from build123d import *

# Parameters (mm, degrees)
F0_R     = 2.794
F1_DEPTH = 2.38125


with BuildPart() as f1:
    # F0 (on Front) → F1 (new body, symmetric)
    with BuildSketch(Plane.XZ):
        with BuildLine():
            ThreePointArc((13.787585, 45.968807), (0, 53.975), (-13.787585, 45.968807))
            Line((-13.787585, 45.968807), (-36.430068, 6.295045))
            ThreePointArc((-36.430068, 6.295045), (-38.1, 0), (-36.430068, -6.295045))
            Line((-36.430068, -6.295045), (-13.787585, -45.968807))
            ThreePointArc((-13.787585, -45.968807), (0, -53.975), (13.787585, -45.968807))
            Line((13.787585, -45.968807), (36.430068, -6.295045))
            ThreePointArc((36.430068, -6.295045), (38.1, 0), (36.430068, 6.295045))
            Line((36.430068, 6.295045), (13.787585, 45.968807))
        make_face()
        with Locations((0, -44.45)):
            Circle(F0_R, mode=Mode.SUBTRACT)
        with Locations((0, 44.45)):
            Circle(F0_R, mode=Mode.SUBTRACT)
    extrude(amount=F1_DEPTH, both=True)


solid = f1.part
Work out the finished part from the listing and answer in its coordinate system (mm). Coordinates: 2 decimals unless noted, no trailing zeros. Order: outer loops, then holes, each group sorted by start corner. A loop starts at its lowest first (then second) coordinate and runs counter-clockwise, first axis right, second up. Notation, with made-up numbers: (62, 84.25) - (68, 84.25) arc R36 cw to (68, 123.25) - close; hole circle Ø7 at (3, 65.25). An arc over 180 degrees is marked (long way). Put each result on its own line as item: value. Start each with the question number.
1) Find section D-D (z = 27.5). Give the vertices of the cut face in (x, y).
2) Find section A-A (x = 0). Give the vertices of the cut face in (y, z) (3 decimals).
3) Find the intervals of material crossed by line 1 (Z direction, x = 0, y = -0.3) (3 decimals); line 2 (Z direction, x = -2, y = 0.5); line 3 (Z direction, x = 7.5, y = -0.9), in increasing order. Write a range as from..to.
4) Find section C-C (z = 44.45). Give the vertices of the cut face in (x, y), plus the area to 3 significant figures.
5) Find section B-B (y = -1.35). Give the vertices of the cut face in (x, z) (3 decimals), plus the area to 3 significant figures.
6) For a pull along Z with two mould halves and no side action, classify faces 1 (the flat face through (-25.27, -0.03, -25.85)), 2 (the cylindrical face through (-0.36, 0.03, -41.68)), 3 (the flat face through (-1, 2.381, 1)) as released by +Z, released by -Z, zero draft, split by the parting line, or undercut.
7) Flat-ended cylindrical pins translate along their axes: pin 1 (1 mm diameter, centred on x = -22.5, y = -2, fed in from +Z); pin 2 (1 mm diameter, centred on y = -1.5, z = 24.5, fed in from +X). Find the tip coordinate at first contact, or state that the pin passes through.
Results list:
1. outline: (-24.33, -2.38) - (24.33, -2.38) - (24.33, 2.38) - (-24.33, 2.38) - close
2. outline: (-2.381, -53.975) - (2.381, -53.975) - (2.381, -47.244) - (-2.381, -47.244) - close; (-2.381, -41.656) - (2.381, -41.656) - (2.381, 41.656) - (-2.381, 41.656) - close; (-2.381, 47.244) - (2.381, 47.244) - (2.381, 53.975) - (-2.381, 53.975) - close
3. line 1: z = -53.975..-47.244, -41.656..41.656, 47.244..53.975
3. line 2: z = -53.85..-46.4, -42.5..42.5, 46.4..53.85
3. line 3: z = -52.09..52.09
4. outline: (-14.65, -2.38) - (-2.79, -2.38) - (-2.79, 2.38) - (-14.65, 2.38) - close; (2.79, -2.38) - (14.65, -2.38) - (14.65, 2.38) - (2.79, 2.38) - close
4. area: 113 mm^2
5. outline: (-36.43, -6.295) - (-13.788, -45.969) arc R15.875 ccw to (13.788, -45.969) - (36.43, -6.295) arc R12.7 ccw to (36.43, 6.295) - (13.788, 45.969) arc R15.875 ccw to (-13.788, 45.969) - (-36.43, 6.295) arc R12.7 ccw to start; hole circle Ø5.588 at (0, -44.45); hole circle Ø5.588 at (0, 44.45)
5. area: 5,190 mm^2
6. face 1: released by -Z
6. face 2: undercut
6. face 3: zero draft
7. pin 1: stops at z = 31.58
7. pin 2: stops at x = 26.33
